```python
from build123d import *

# Parameters (mm, degrees)
ESBO_O1_R                = 5.5
RESSALTO_EXTRUS_O1_DEPTH = 6
ESBO_O2_W                = 13.5
ESBO_O2_H                = 13.5
RESSALTO_EXTRUS_O2_DEPTH = 6
FILETE1_R                = 8
ESBO_O3_R                = 1.5
CORTE_EXTRUS_O1_DEPTH    = 6
ESBO_O5_R                = 3.5
CORTE_EXTRUS_O2_DEPTH    = 6


with BuildPart() as part:
    # Esboço1 → Ressalto-extrusão1 (new body)
    with BuildSketch(Plane.XY):
        with BuildLine():
            Line((-20, 33.5), (20, 33.5))
            ThreePointArc((20, 33.5), (29.545941546, 29.545941546), (33.5, 20))
            Line((33.5, 20), (33.5, -20))
            ThreePointArc((33.5, -20), (29.545941546, -29.545941546), (20, -33.5))
            Line((20, -33.5), (-20, -33.5))
            ThreePointArc((-20, -33.5), (-29.545941546, -29.545941546), (-33.5, -20))
            Line((-33.5, -20), (-33.5, 20))
            ThreePointArc((-33.5, 20), (-29.545941546, 29.545941546), (-20, 33.5))
        make_face()
        with Locations((-20, 20)):
            Circle(ESBO_O1_R, mode=Mode.SUBTRACT)
        with Locations((20, 20)):
            Circle(ESBO_O1_R, mode=Mode.SUBTRACT)
        with Locations((0, -20)):
            Circle(ESBO_O1_R, mode=Mode.SUBTRACT)
    extrude(amount=RESSALTO_EXTRUS_O1_DEPTH)

    # Esboço2 → Ressalto-extrusão2 (add)
    with BuildSketch(Plane(origin=(0, 0, 0), x_dir=(-1, 0, 0), z_dir=(0, 0, -1))):
        with Locations((-26.75, -26.75)):
            Rectangle(ESBO_O2_W, ESBO_O2_H)
        with Locations((26.75, -26.75)):
            Rectangle(ESBO_O2_W, ESBO_O2_H)
    extrude(amount=-RESSALTO_EXTRUS_O2_DEPTH)

    # Filete1
    filete1_edges = [part.edges().sort_by_distance(p)[0] for p in [
        (33.5, -33.5, 3),
        (-33.5, -33.5, 3),
    ]]
    fillet(filete1_edges, radius=FILETE1_R)

    # Esboço3 → Corte-extrusão1 (cut)
    with BuildSketch(Plane(origin=(0, 0, 0), x_dir=(-1, 0, 0), z_dir=(0, 0, -1))):
        with Locations((0, 20)):
            Circle(ESBO_O3_R)
        with Locations((20, -20)):
            Circle(ESBO_O3_R)
        with Locations((-20, -20)):
            Circle(ESBO_O3_R)
    extrude(amount=-CORTE_EXTRUS_O1_DEPTH, mode=Mode.SUBTRACT)

    # Esboço5 → Corte-extrusão2 (cut)
    with BuildSketch(Plane.XY.offset(6)):
        with Locations((-12, 7)):
            Circle(ESBO_O5_R)
        with Locations((12, 7)):
            Circle(ESBO_O5_R)
    extrude(amount=-CORTE_EXTRUS_O2_DEPTH, mode=Mode.SUBTRACT)


solid = part.part
```
Verification items for the finished model (mm, model axes). Round coordinates to 2 decimals unless told otherwise and drop trailing zeros. Write each loop counter-clockwise with the first axis right and the second up, starting at its lowest first coordinate (ties: lowest second). Pieces come first, ordered by that corner, then holes.
1. Section check A-A on y = -20. Enter the section's corners in (x, z).
2. Section check B-B on z = 1.4. State how many separate pieces and enclosed holes the cut face has, plus the area to 3 significant figures.
3. Draft check along X on faces 1 (the cylindrical face through (-12.759, 3.583, 3.042)), 2 (the flat face through (0, 0, 0)), 3 (the cylindrical face through (29.44, 29.65, 2.96)). Enter one of: +X half, -X half, draft (parallel to the pull), parting line (faces both ways), or undercut.
4. Gauge pin test, flat end, axial feed: P1, Ø2.5, axis at x = 20, y = -20, coming from the +Z side (3 decimals). Record the tip position at first contact, or that the pin passes through.
5. Scan lines: L1, parallel to Y at x = 20, z = 4.7; L2, parallel to X at y = 8.5, z = 3.3; L3, parallel to X at y = 18, z = 4.65. Record each from-to range of solid material in increasing order.
6. Section check D-D on y = 15.5. Enter the section's corners in (x, z).
7. Section check C-C on x = 4.5. Enter the section's corners in (y, z), plus the area to 3 significant figures.
Answer:
1. outline: (-33.5, 0) - (-21.5, 0) - (-21.5, 6) - (-33.5, 6) - close; (-18.5, 0) - (-5.5, 0) - (-5.5, 6) - (-18.5, 6) - close; (5.5, 0) - (18.5, 0) - (18.5, 6) - (5.5, 6) - close; (21.5, 0) - (33.5, 0) - (33.5, 6) - (21.5, 6) - close
2. separate pieces: 1
2. enclosed holes: 8
2. area: 4,000 mm2
3. face 1: undercut
3. face 2: draft
3. face 3: +X half
4. P1: passes through
5. L1: y = -33.5 to -21.5, -18.5 to 14.5, 25.5 to 33.5
5. L2: x = -33.5 to -15.16, -8.84 to 8.84, 15.16 to 33.5
5. L3: x = -33.5 to -25.12, -14.88 to 14.88, 25.12 to 33.5
6. outline: (-33.5, 0) - (-23.16, 0) - (-23.16, 6) - (-33.5, 6) - close; (-16.84, 0) - (16.84, 0) - (16.84, 6) - (-16.84, 6) - close; (23.16, 0) - (33.5, 0) - (33.5, 6) - (23.16, 6) - close
7. outline: (-33.5, 0) - (-23.16, 0) - (-23.16, 6) - (-33.5, 6) - close; (-16.84, 0) - (33.5, 0) - (33.5, 6) - (-16.84, 6) - close
7. area: 364 mm2
